Design review of the part built by this model. Coordinates are the model's own, in mm. Face numbers are marked on the shaded views. A direction names the side the tool comes from. Round coordinates to 2 decimals unless told otherwise and drop trailing zeros. Order: outer loops, then holes, each group sorted by start corner. A loop starts at its lowest first (then second) coordinate and runs counter-clockwise, first axis right, second up.
from build123d import *

# Parameters (mm, degrees)
F1_R      = 10.668
F3_R      = 7.8994
F4_DEPTH  = 23.6982
F5_R      = 7.8994
F6_DEPTH  = 23.6982
F7_SIZE   = 2
F8_R      = 7.8994
F8_R_2    = 7.6494
F9_DEPTH  = 23.6982
F10_R     = 7.8994
F10_R_2   = 7.6494
F11_DEPTH = 23.6982


with BuildPart() as f2:
    # F2: sweep along a path in F0
    with BuildLine(Plane.YZ) as f2_path:
        ThreePointArc((0, 0), (-8.7867965644, 21.2132034356), (-30, 30))
    # F1 (on Top) → F2 (sweep)
    with BuildSketch(Plane.XY):
        Circle(F1_R)
    sweep(path=f2_path.line)

    # F3 (on face) → F4 (join)
    with BuildSketch(Plane(origin=(0, 0, 0), x_dir=(1, 0, 0), z_dir=(0, 0, -1))):
        Circle(F3_R)
    extrude(amount=F4_DEPTH)

    # F5 (on face) → F6 (join)
    with BuildSketch(Plane.XZ.offset(30)):
        with Locations((0, 30)):
            Circle(F5_R)
    extrude(amount=F6_DEPTH)

    # F7
    f7_edges = [f2.edges().sort_by_distance(p)[0] for p in [
        (-7.8994, 0, -23.6982),
        (-7.8994, -53.6982, 30),
    ]]
    chamfer(f7_edges, length=F7_SIZE)

    # F8 (on face) → F9 (cut, through all)
    with BuildSketch(Plane(origin=(0, 0, -23.6982), x_dir=(1, 0, 0), z_dir=(0, 0, -1))):
        Circle(F8_R)
        Circle(F8_R_2, mode=Mode.SUBTRACT)
    extrude(amount=-F9_DEPTH, mode=Mode.SUBTRACT)

    # F10 (on face) → F11 (cut, through all)
    with BuildSketch(Plane.XZ.offset(53.6982)):
        with Locations((0, 30)):
            Circle(F10_R)
        with Locations((0, 30)):
            Circle(F10_R_2, mode=Mode.SUBTRACT)
    extrude(amount=-F11_DEPTH, mode=Mode.SUBTRACT)


solid = f2.part
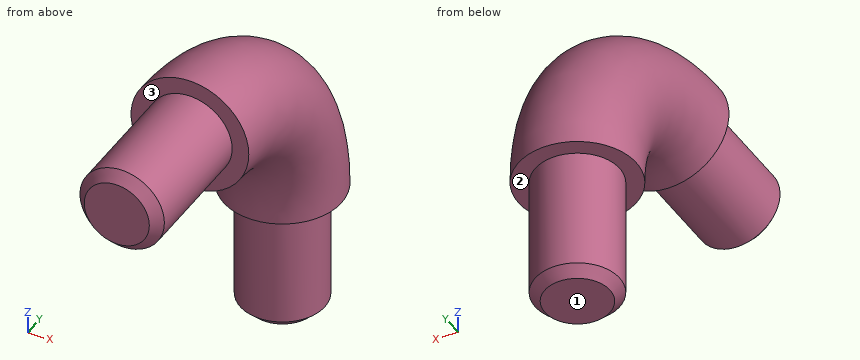
1) Take a section at C-C on z = -12. Give the boundary of the cut face in (x, y), plus the area to 3 significant figures.
Results:
outline: circle Ø15.3 at (0, 0)
area: 184 mm2
2) Clearance check with flat-ended pins moving along their axes: P1, Ø1, axis at x = 2.5, y = -14, coming from the +Z side; P2, Ø3, axis at x = 5.5, y = -10.5, coming from the -Z side; P3, Ø5, axis at y = -29, z = 21.5, coming from the -X side. State where each tip first meets the part, or that it passes through.
Results:
P1: stops at z = 37.31
P2: stops at z = 0
P3: stops at x = -8.84
3) Take a section at A-A on x = 0. Give the boundary of the cut face in (y, z), plus the area to 3 significant figures.
Results:
outline: (-53.7, 24.1) - (-51.95, 22.35) - (-30, 22.35) - (-30, 19.33) arc R19.33 cw to (-10.67, 0) - (-7.65, 0) - (-7.65, -21.95) - (-5.9, -23.7) - (5.9, -23.7) - (7.65, -21.95) - (7.65, 0) - (10.67, 0) arc R40.67 ccw to (-30, 40.67) - (-30, 37.65) - (-51.95, 37.65) - (-53.7, 35.9) - close
area: 1,720 mm2
4) To check wall thickness, follow line 1 along Y through (x, z) = (3, -2); line 2 along Y through (x, z) = (-5.75, -13); line 3 along X through (y, z) = (-1, -16.5). State the ranges of each line that lie inside material, in increasing order.
Results:
line 1: y = -7.04 to 7.04
line 2: y = -5.04 to 5.04
line 3: x = -7.58 to 7.58
5) Take a section at B-B on y = -38.5. Give the boundary of the cut face in (x, z), plus the area to 3 significant figures.
Results:
outline: circle Ø15.3 at (0, 30)
area: 184 mm2
6) For the marked faces 1, 2 and 3, list the 3-axis set-ups (+Z, -Z, +X, -X, +Y, -Y) from which the entire face can be reached by the end or side of a thin tool; tool diameter is ignored.
Results:
face 1: -Z, +X, -X, +Y, -Y
face 2: -Z
face 3: -Y
